For this review, take the finished solid that the model builds, in its own axes (mm). Face numbers are marked on the shaded views. A direction names the side the tool comes from. Coordinates: 2 decimals unless noted, no trailing zeros. Order: outer loops, then holes, each group sorted by start corner. A loop starts at its lowest first (then second) coordinate and runs counter-clockwise, first axis right, second up. Notation, with made-up numbers: M 51.5,52 L 97.5,52 A17 ccw 97.5,78 Z; hole C 59.25,52 d7. An arc over 180 degrees is marked long. Use CSV: the item, a comma, the result in double quotes.
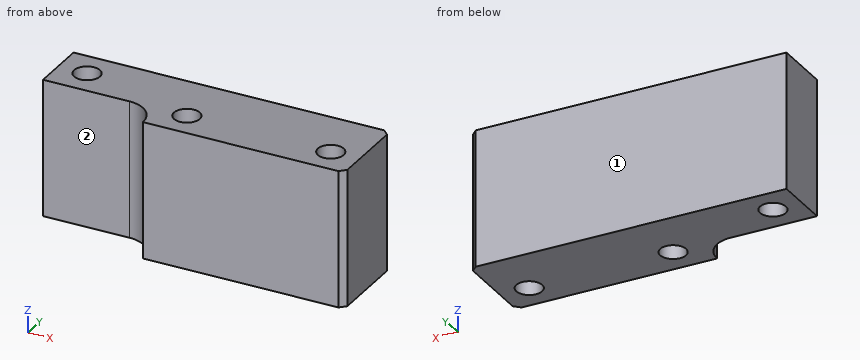
```python
from build123d import *

# Parameters (mm, degrees)
SKETCH_1_R      = 4.5
EXTRUDE_1_DEPTH = 47.5
FILLET_1_R      = 10
CHAMFER_1_SIZE  = 2


with BuildPart() as part:
    # 草图1 → 凸台-拉伸1 (new body)
    with BuildSketch(Plane.XY):
        Polygon((-35, 0), (-35, -10), (35, -10), (35, 10), (35, 20), (-35, 20), (-65, 20), (-75, 20), (-75, 0), align=None)
        with Locations((-25, 0)):
            Circle(SKETCH_1_R, mode=Mode.SUBTRACT)
        with Locations((25, 0)):
            Circle(SKETCH_1_R, mode=Mode.SUBTRACT)
        with Locations((-65, 10)):
            Circle(SKETCH_1_R, mode=Mode.SUBTRACT)
    extrude(amount=EXTRUDE_1_DEPTH)

    # 圆角1
    fillet_1_edges = [part.edges().sort_by_distance(p)[0] for p in [
        (-35, 0, 23.75),
    ]]
    fillet(fillet_1_edges, radius=FILLET_1_R - 0.0001)  # a hair under: the kernel refuses the full size

    # 倒角1
    chamfer_1_edges = [part.edges().sort_by_distance(p)[0] for p in [
        (35, -10, 23.75),
        (35, 20, 23.75),
    ]]
    chamfer(chamfer_1_edges, length=CHAMFER_1_SIZE)


solid = part.part
```
Item 1: Add section B-B on y = 10. State the section outline as (x, z) points, and give its area (3 significant figures).
Solutions:
outline,"M -75,0 L -69.5,0 L -69.5,47.5 L -75,47.5 Z; M -60.5,0 L 35,0 L 35,47.5 L -60.5,47.5 Z"
area,"4,800 mm^2"
Item 2: Clearance check with flat-ended pins moving along their axes: pin 1 Ø8 at (x, y) = (5, 6.5) entering from -Z; pin 2 Ø9 at (x, z) = (-58.5, 35.5) entering from -Y; pin 3 Ø1.5 at (x, z) = (-37, 34.5) entering from -Y. State where each tip first meets the part, or that it passes through.
Solutions:
pin 1,"z = 0"
pin 2,"y = 0"
pin 3,"y = -5.16"
Item 3: To check wall thickness, follow line 1 along Y through (x, z) = (25, 13); line 2 along Y through (x, z) = (-65, 10); line 3 along X through (y, z) = (-1.5, 7). State the ranges of each line that lie inside material, in increasing order. Write a range as [from, to].
Solutions:
line 1,"[-10, -4.5], [4.5, 20]"
line 2,"[0, 5.5], [14.5, 20]"
line 3,"[-39.73, -29.24], [-20.76, 20.76], [29.24, 35]"
Item 4: Add section C-C on z = 17. State how many separate pieces and enclosed holes the cut face has, and give its area (3 significant figures).
Solutions:
separate pieces,"1"
enclosed holes,"3"
area,"2,730 mm^2"
Item 5: For the marked faces 1 and 2, list the 3-axis set-ups (+Z, -Z, +X, -X, +Y, -Y) from which the entire face can be reached by the end or side of a thin tool; tool diameter is ignored.
Solutions:
face 1,"+Z, -Z, +X, -X, +Y"
face 2,"+Z, -Z, -X, -Y"
Item 6: Add section A-A on x = -65. State the section outline as (y, z) points, and give its area (4 significant figures).
Solutions:
outline,"M 0,0 L 5.5,0 L 5.5,47.5 L 0,47.5 Z; M 14.5,0 L 20,0 L 20,47.5 L 14.5,47.5 Z"
area,"522.5 mm^2"
Item 7: Add section D-D on x = -51.5. State the section outline as (y, z) points.
Solutions:
outline,"M 0,0 L 20,0 L 20,47.5 L 0,47.5 Z"
